from build123d import *

# Parameters (mm, degrees)
SKETCH1_R           = 12.811295034
SKETCH1_R_2         = 19.687662737
BOSS_EXTRUDE1_DEPTH = 254
CUT_EXTRUDE1_DEPTH  = 241.3


with BuildPart() as part:
    # Sketch1 → Boss-Extrude1 (new body)
    with BuildSketch(Plane(origin=(0, 0, 0), x_dir=(1, 0, 0), z_dir=(0, 1, 0))):
        with BuildLine():
            Line((-133.764264849, 68.038364167), (348.835735151, 68.038364167))
            ThreePointArc((348.835735151, 68.038364167), (357.815991272, 64.318620289), (361.535735151, 55.338364167))
            Line((361.535735151, 55.338364167), (361.535735151, -173.261635833))
            ThreePointArc((361.535735151, -173.261635833), (357.815991272, -182.241891954), (348.835735151, -185.961635833))
            Line((348.835735151, -185.961635833), (-133.764264849, -185.961635833))
            ThreePointArc((-133.764264849, -185.961635833), (-142.74452097, -182.241891954), (-146.464264849, -173.261635833))
            Line((-146.464264849, -173.261635833), (-146.464264849, 55.338364167))
            ThreePointArc((-146.464264849, 55.338364167), (-142.74452097, 64.318620289), (-133.764264849, 68.038364167))
        make_face()
        with Locations((107.535735151, 48.988364167)):
            Circle(SKETCH1_R, mode=Mode.SUBTRACT)
        with Locations((107.535735151, -69.423369036)):
            Circle(SKETCH1_R_2, mode=Mode.SUBTRACT)
    extrude(amount=-BOSS_EXTRUDE1_DEPTH)

    # Sketch2 → Cut-Extrude1 (cut)
    with BuildSketch(Plane(origin=(0, 0, 0), x_dir=(1, 0, 0), z_dir=(0, 1, 0))):
        with BuildLine():
            Line((-108.364264849, 29.938364167), (323.435735151, 29.938364167))
            ThreePointArc((323.435735151, 29.938364167), (332.415991272, 26.218620289), (336.135735151, 17.238364167))
            Line((336.135735151, 17.238364167), (336.135735151, -147.861635833))
            ThreePointArc((336.135735151, -147.861635833), (332.415991272, -156.841891954), (323.435735151, -160.561635833))
            Line((323.435735151, -160.561635833), (-108.364264849, -160.561635833))
            ThreePointArc((-108.364264849, -160.561635833), (-117.34452097, -156.841891954), (-121.064264849, -147.861635833))
            Line((-121.064264849, -147.861635833), (-121.064264849, 17.238364167))
            ThreePointArc((-121.064264849, 17.238364167), (-117.34452097, 26.218620289), (-108.364264849, 29.938364167))
        make_face()
    extrude(amount=-CUT_EXTRUDE1_DEPTH, mode=Mode.SUBTRACT)


solid = part.part
Could you check a few things on this model? Use its own coordinates, in mm. A direction names the side the tool comes from. Round coordinates to 2 decimals unless told otherwise and drop trailing zeros. Order: outer loops, then holes, each group sorted by start corner. A loop starts at its lowest first (then second) coordinate and runs counter-clockwise, first axis right, second up.
(1) Imagine slicing it at A-A (x = -11). Write out the boundary of the cut face in (y, z).
Response values:
outline: (-254, -68.04) - (0, -68.04) - (0, -29.94) - (-241.3, -29.94) - (-241.3, 160.56) - (0, 160.56) - (0, 185.96) - (-254, 185.96) - close
(2) If we mould it in two halves opening along Z, with no side actions, what happens to faces 3 (the flat face through (111, -241.3, 43)), 4 (the cylindrical face through (357.914, -125.222, 182.143)), 5 (the flat face through (-121.064, -119, 66)), 6 (the flat face through (-146.464, -125, 61))? For each: released by +Z, released by -Z, zero draft, split by the parting line, or undercut.
Response values:
face 3: undercut
face 4: released by +Z
face 5: undercut
face 6: zero draft
(3) I'm going to push a flat-ended pin straight in: pin 1 (1.5 mm diameter, centred on x = 6, z = 12.5, fed in from +Y). Where does the tip first touch, or does it pass through?
Response values:
pin 1: stops at y = -241.3
(4) Please list where these lines run through material, in increasing order: line 1 along Z through (x, y) = (286, -61); line 2 along X through (y, z) = (-233.5, 138.5); line 3 along Z through (x, y) = (103.5, -224).
Response values:
line 1: z = -68.04 to -29.94, 160.56 to 185.96
line 2: x = -146.46 to -121.06, 336.14 to 361.54
line 3: z = -68.04 to -61.15, -36.83 to -29.94, 160.56 to 185.96
(5) Imagine slicing it at C-C (y = -64.5). Write out the boundary of the cut face in (x, z), plus the area to 3 significant figures.
Response values:
outline: (-146.46, -55.34) arc R12.7 ccw to (-133.76, -68.04) - (348.84, -68.04) arc R12.7 ccw to (361.54, -55.34) - (361.54, 173.26) arc R12.7 ccw to (348.84, 185.96) - (-133.76, 185.96) arc R12.7 ccw to (-146.46, 173.26) - close; hole (-121.06, -17.24) arc R12.7 ccw to (-108.36, -29.94) - (323.44, -29.94) arc R12.7 ccw to (336.14, -17.24) - (336.14, 147.86) arc R12.7 ccw to (323.44, 160.56) - (-108.36, 160.56) arc R12.7 ccw to (-121.06, 147.86) - close; hole circle Ø25.62 at (107.54, -48.99)
area: 41,400 mm2
(6) Imagine slicing it at B-B (z = 97.5). Write out the boundary of the cut face in (x, y).
Response values:
outline: (-146.46, -254) - (361.54, -254) - (361.54, 0) - (336.14, 0) - (336.14, -241.3) - (-121.06, -241.3) - (-121.06, 0) - (-146.46, 0) - close
(7) Which directions (+Z, -Z, +X, -X, +Y, -Y) give clear straight access to the entire face, cutting with the end or side of a thin tool? Please do faces 1 (the flat face through (111, -119, 160.562)), 2 (the flat face through (111, -125, 185.962)).
Response values:
face 1: +Y
face 2: +Z, +X, -X, +Y, -Y
